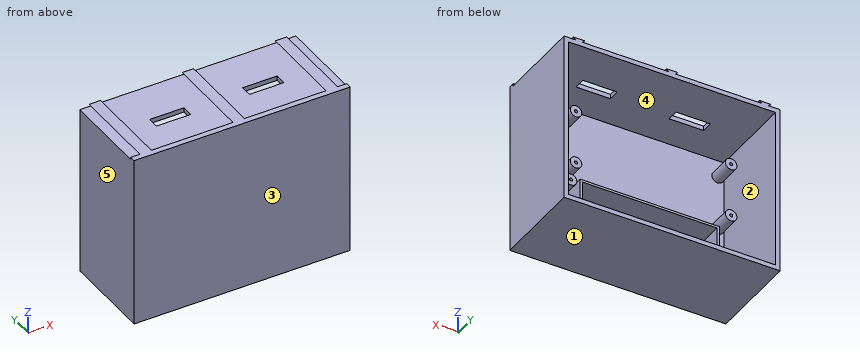
```python
from build123d import *

# Parameters (mm, degrees)
SZKIC1_W                    = 180
SZKIC1_H                    = 140
DODANIE_WYCI_GNI_CIE1_DEPTH = 4
SZKIC6_R                    = 5
SZKIC6_R_2                  = 1.35
DODANIE_WYCI_GNI_CIE2_DEPTH = 20
SZKIC13_W                   = 188
SZKIC13_H                   = 148
SZKIC13_W_2                 = 180
SZKIC13_H_2                 = 140
DODANIE_WYCI_GNI_CIE3_DEPTH = 80
SZKIC14_W                   = 188
SZKIC14_H                   = 5
DODANIE_WYCI_GNI_CIE4_DEPTH = 2
DODANIE_WYCI_GNI_CIE5_DEPTH = 75
WYTNIJ_WYCI_GNI_CIE1_REACH  = 352.281
SZKIC17_W                   = 30
SZKIC17_H                   = 10


with BuildPart() as part:
    # Szkic1 → Dodanie-wyciągnięcie1 (new body)
    with BuildSketch(Plane(origin=(0, 0, 0), x_dir=(-1, 0, 0), z_dir=(0, 1, 0))):
        with Locations((-213.234437894, 908.204921089)):
            Rectangle(SZKIC1_W, SZKIC1_H)
    extrude(amount=DODANIE_WYCI_GNI_CIE1_DEPTH)

    # Szkic6 → Dodanie-wyciągnięcie2 (add)
    # profile 1 of 8: a face of its own
    with BuildSketch(Plane(origin=(0, 4, 0), x_dir=(1, 0, 0), z_dir=(0, 1, 0))):
        with Locations(Location((263.804943957, -915.877316695, 0), (0, 0, 270))):
            Circle(SZKIC6_R)
        with Locations(Location((263.804943957, -915.877316695, 0), (0, 0, 270))):
            Circle(SZKIC6_R_2, mode=Mode.SUBTRACT)
    # profile 2 of 8: a face of its own
    with BuildSketch(Plane(origin=(0, 4, 0), x_dir=(1, 0, 0), z_dir=(0, 1, 0))):
        with Locations(Location((263.804943957, -962.877316695, 0), (0, 0, 270))):
            Circle(SZKIC6_R)
        with Locations(Location((263.804943957, -962.877316695, 0), (0, 0, 270))):
            Circle(SZKIC6_R_2, mode=Mode.SUBTRACT)
    # profile 3 of 8: a face of its own
    with BuildSketch(Plane(origin=(0, 4, 0), x_dir=(1, 0, 0), z_dir=(0, 1, 0))):
        with Locations(Location((128.804943957, -915.877316695, 0), (0, 0, 270))):
            Circle(SZKIC6_R)
        with Locations(Location((128.804943957, -915.877316695, 0), (0, 0, 270))):
            Circle(SZKIC6_R_2, mode=Mode.SUBTRACT)
    # profile 4 of 8: a face of its own
    with BuildSketch(Plane(origin=(0, 4, 0), x_dir=(1, 0, 0), z_dir=(0, 1, 0))):
        with Locations(Location((128.804943957, -962.877316695, 0), (0, 0, 270))):
            Circle(SZKIC6_R)
        with Locations(Location((128.804943957, -962.877316695, 0), (0, 0, 270))):
            Circle(SZKIC6_R_2, mode=Mode.SUBTRACT)
    # profile 5 of 8: a face of its own
    with BuildSketch(Plane(origin=(0, 4, 0), x_dir=(1, 0, 0), z_dir=(0, 1, 0))):
        with Locations(Location((268.102028807, -898.653399162, 0), (0, 0, 270))):
            Circle(SZKIC6_R)
        with Locations(Location((268.102028807, -898.653399162, 0), (0, 0, 270))):
            Circle(SZKIC6_R_2, mode=Mode.SUBTRACT)
    # profile 6 of 8: a face of its own
    with BuildSketch(Plane(origin=(0, 4, 0), x_dir=(1, 0, 0), z_dir=(0, 1, 0))):
        with Locations(Location((295.102028807, -898.653399162, 0), (0, 0, 270))):
            Circle(SZKIC6_R)
        with Locations(Location((295.102028807, -898.653399162, 0), (0, 0, 270))):
            Circle(SZKIC6_R_2, mode=Mode.SUBTRACT)
    # profile 7 of 8: a face of its own
    with BuildSketch(Plane(origin=(0, 4, 0), x_dir=(1, 0, 0), z_dir=(0, 1, 0))):
        Polygon((258.182980941, -864.357234477), (260.182980941, -864.357234477), (260.182980941, -839.857234477), (139.182980941, -839.857234477), (139.182980941, -863.857234467), (141.182980941, -863.857234467), (141.182980941, -841.857234452), (258.182980941, -841.857234452), align=None)
    # profile 8 of 8: a face of its own
    with BuildSketch(Plane(origin=(0, 4, 0), x_dir=(1, 0, 0), z_dir=(0, 1, 0))):
        Polygon((141.182980941, -877.857234487), (141.182980941, -899.857234503), (258.182980941, -899.857234503), (258.182980941, -877.357234477), (260.182980941, -877.357234477), (260.182980941, -901.857234477), (139.182980941, -901.857234477), (139.182980941, -877.857234487), align=None)
    extrude(amount=DODANIE_WYCI_GNI_CIE2_DEPTH)

    # Szkic13 → Dodanie-wyciągnięcie3 (add)
    with BuildSketch(Plane.XZ):
        with Locations((213.234437894, 908.204921089)):
            Rectangle(SZKIC13_W, SZKIC13_H)
        with Locations((213.234437894, 908.204921089)):
            Rectangle(SZKIC13_W_2, SZKIC13_H_2, mode=Mode.SUBTRACT)
    extrude(amount=-DODANIE_WYCI_GNI_CIE3_DEPTH)

    # Szkic14 → Dodanie-wyciągnięcie4 (add)
    with BuildSketch(Plane.XY.offset(982.204921089)):
        with Locations((213.234437894, 2.5)):
            Rectangle(SZKIC14_W, SZKIC14_H)
    extrude(amount=DODANIE_WYCI_GNI_CIE4_DEPTH)

    # Szkic15 → Dodanie-wyciągnięcie5 (add)
    with BuildSketch(Plane(origin=(0, 5, 0), x_dir=(1, 0, 0), z_dir=(0, 1, 0))):
        Polygon((299.287557022, -984.204921089), (297.234437894, -982.204921089), (291.287557022, -982.204921089), (289.287557022, -984.204921089), align=None)
        Polygon((135.234437894, -982.204921089), (129.234437894, -982.204921089), (127.234437894, -984.204921089), (137.234437894, -984.204921089), align=None)
        Polygon((208.260997458, -984.204921089), (218.260997458, -984.204921089), (216.260997458, -982.204921089), (210.260997458, -982.204921089), align=None)
    extrude(amount=DODANIE_WYCI_GNI_CIE5_DEPTH)

    # Szkic17 → Wytnij-wyciągnięcie1 (cut, up to next)
    with BuildSketch(Plane.XY.offset(982.204921089), mode=Mode.PRIVATE) as wytnij_wyci_gni_cie1_sk1:
        with Locations((253.77427724, 37.5)):
            Rectangle(SZKIC17_W, SZKIC17_H)
    wytnij_wyci_gni_cie1_tool1 = extrude(wytnij_wyci_gni_cie1_sk1.sketch, amount=-WYTNIJ_WYCI_GNI_CIE1_REACH, mode=Mode.PRIVATE) & part.part
    # Szkic17 → Wytnij-wyciągnięcie1 (cut, up to next)
    with BuildSketch(Plane.XY.offset(982.204921089), mode=Mode.PRIVATE) as wytnij_wyci_gni_cie1_sk2:
        with Locations((172.747717676, 37.5)):
            Rectangle(SZKIC17_W, SZKIC17_H)
    wytnij_wyci_gni_cie1_tool2 = extrude(wytnij_wyci_gni_cie1_sk2.sketch, amount=-WYTNIJ_WYCI_GNI_CIE1_REACH, mode=Mode.PRIVATE) & part.part
    add(wytnij_wyci_gni_cie1_tool1.solids().sort_by_distance((253.774277, 37.5, 982.204921))[0], mode=Mode.SUBTRACT)
    add(wytnij_wyci_gni_cie1_tool2.solids().sort_by_distance((172.747718, 37.5, 982.204921))[0], mode=Mode.SUBTRACT)


solid = part.part
```
Geometry check sheet. Reference: the model listing, model coordinates, mm. Face numbers are marked on the shaded views. A direction names the side the tool comes from. Give positions to 0.01 mm unless a question says otherwise; leave off trailing zeros. Write each loop counter-clockwise with the first axis right and the second up, starting at its lowest first coordinate (ties: lowest second). Pieces come first, ordered by that corner, then holes. Notation, with made-up numbers: (41.25, -2) - (59.25, -2) arc R21 ccw to (59.25, 35) - close; hole circle Ø4 at (38.25, -25). An arc over 180 degrees is marked (long way). Use a Markdown table: item, result.
Q1. Thickness scan on L1, parallel to Z at x = 161, y = 6.5; L2, parallel to X at y = 71, z = 929; L3, parallel to X at y = 16.5, z = 903. Record the ranges inside material, lowest first. Write a range as [from, to].
Computed:
| item | result |
|---|---|
| L1 | z = [834.2, 838.2], [839.86, 841.86], [899.86, 901.86], [978.2, 982.2] |
| L2 | x = [119.23, 123.23], [303.23, 307.23] |
| L3 | x = [119.23, 123.23], [265.63, 270.57], [292.63, 297.57], [303.23, 307.23] |
Q2. Go/stop test with flat-tipped pins: P1, Ø5, axis at x = 265.5, z = 963.5, coming from the +Y side; P2, Ø3, axis at x = 185, y = 12.5, coming from the +Z side; P3, Ø2, axis at x = 301.5, z = 983.5, coming from the +Y side. Record where each tip stops, or that it passes through.
Computed:
| item | result |
|---|---|
| P1 | stops at y = 24 |
| P2 | stops at z = 982.2 |
| P3 | stops at y = 5 |
Q3. Draft check along Z on the marked faces 1, 2 and 3. Enter one of: pulls with the +Z half, pulls with the -Z half, needs draft (parallel to the pull), parting line crosses it, or undercut.
Computed:
| item | result |
|---|---|
| face 1 | pulls with the -Z half |
| face 2 | undercut |
| face 3 | needs draft |
Q4. Section check C-C, the plane y = 40. Enter the section's corners in (x, z).
Computed:
| item | result |
|---|---|
| outline | (119.23, 834.2) - (307.23, 834.2) - (307.23, 982.2) - (297.23, 982.2) - (299.29, 984.2) - (289.29, 984.2) - (291.29, 982.2) - (268.77, 982.2) - (268.77, 978.2) - (303.23, 978.2) - (303.23, 838.2) - (123.23, 838.2) - (123.23, 978.2) - (157.75, 978.2) - (157.75, 982.2) - (135.23, 982.2) - (137.23, 984.2) - (127.23, 984.2) - (129.23, 982.2) - (119.23, 982.2) - close; (187.75, 978.2) - (238.77, 978.2) - (238.77, 982.2) - (216.26, 982.2) - (218.26, 984.2) - (208.26, 984.2) - (210.26, 982.2) - (187.75, 982.2) - close |
Q5. Set-up check for the marked faces 4 and 5: record each of +Z, -Z, +X, -X, +Y, -Y from which the full face is reachable in a straight line by a thin tool's end or side.
Computed:
| item | result |
|---|---|
| face 4 | +Y |
| face 5 | +Z, -Z, -X, +Y, -Y |
Q6. Section check A-A, the plane x = 249.5. Enter the section's corners in (y, z).
Computed:
| item | result |
|---|---|
| outline | (0, 834.2) - (80, 834.2) - (80, 838.2) - (4, 838.2) - (4, 839.86) - (24, 839.86) - (24, 841.86) - (4, 841.86) - (4, 899.86) - (24, 899.86) - (24, 901.86) - (4, 901.86) - (4, 978.2) - (32.5, 978.2) - (32.5, 982.2) - (5, 982.2) - (5, 984.2) - (0, 984.2) - close; (42.5, 978.2) - (80, 978.2) - (80, 982.2) - (42.5, 982.2) - close |
Q7. Section check B-B, the plane y = 55. Enter the section's corners in (x, z), then the cut area to 3 significant figures.
Computed:
| item | result |
|---|---|
| outline | (119.23, 834.2) - (307.23, 834.2) - (307.23, 982.2) - (297.23, 982.2) - (299.29, 984.2) - (289.29, 984.2) - (291.29, 982.2) - (216.26, 982.2) - (218.26, 984.2) - (208.26, 984.2) - (210.26, 982.2) - (135.23, 982.2) - (137.23, 984.2) - (127.23, 984.2) - (129.23, 982.2) - (119.23, 982.2) - close; hole (123.23, 838.2) - (303.23, 838.2) - (303.23, 978.2) - (123.23, 978.2) - close |
| area | 2,670 mm² |
Q8. Section check D-D, the plane z = 871. Enter the section's corners in (x, y), then the cut area to 3 significant figures.
Computed:
| item | result |
|---|---|
| outline | (119.23, 0) - (307.23, 0) - (307.23, 80) - (303.23, 80) - (303.23, 4) - (123.23, 4) - (123.23, 80) - (119.23, 80) - close |
| area | 1,360 mm² |
